```python
from build123d import *

# Parameters (mm, degrees)
ESQUISSE1_W             = 40
ESQUISSE1_H             = 27
ESQUISSE1_W_2           = 37
ESQUISSE1_H_2           = 24
BOSS_EXTRU_1_DEPTH      = 300
ESQUISSE2_R             = 2.5
ENL_V_MAT_EXTRU_1_DEPTH = 304.856874202
ESQUISSE3_R             = 6
ESQUISSE3_R_2           = 2.75
ESQUISSE3_R_3           = 10
ENL_V_MAT_EXTRU_2_DEPTH = 304.856874202


with BuildPart() as part:
    # Esquisse1 → Boss.-Extru.1 (new body)
    with BuildSketch(Plane.XY):
        with Locations((20, 13.5)):
            Rectangle(ESQUISSE1_W, ESQUISSE1_H)
        with Locations((20, 13.5)):
            Rectangle(ESQUISSE1_W_2, ESQUISSE1_H_2, mode=Mode.SUBTRACT)
    extrude(amount=BOSS_EXTRU_1_DEPTH)

    # Esquisse2 → Enlèv. mat.-Extru.1 (cut, through all)
    with BuildSketch(Plane(origin=(0, 0, 0), x_dir=(1, 0, 0), z_dir=(0, 1, 0))):
        with Locations(Location((8, -290, 0), (0, 0, 90))):
            Circle(ESQUISSE2_R)
        with Locations(Location((32, -258, 0), (0, 0, 90))):
            Circle(ESQUISSE2_R)
        with Locations(Location((7, -258, 0), (0, 0, 90))):
            Circle(ESQUISSE2_R)
        with Locations(Location((31, -290, 0), (0, 0, 90))):
            Circle(ESQUISSE2_R)
    extrude(amount=ENL_V_MAT_EXTRU_1_DEPTH, mode=Mode.SUBTRACT)

    # Esquisse3 → Enlèv. mat.-Extru.2 (cut, through all)
    with BuildSketch(Plane(origin=(0, 0, 0), x_dir=(1, 0, 0), z_dir=(0, 1, 0))):
        with Locations(Location((20, -30, 0), (0, 0, 90))):
            Circle(ESQUISSE3_R)
        with Locations(Location((5, -15, 0), (0, 0, 90))):
            Circle(ESQUISSE3_R_2)
        with Locations(Location((20, -100, 0), (0, 0, 90))):
            Circle(ESQUISSE3_R_3)
        with Locations(Location((35, -15, 0), (0, 0, 90))):
            Circle(ESQUISSE3_R_2)
        with Locations(Location((35, -45, 0), (0, 0, 90))):
            Circle(ESQUISSE3_R_2)
        with Locations(Location((5, -45, 0), (0, 0, 90))):
            Circle(ESQUISSE3_R_2)
        with Locations(Location((5, -185, 0), (0, 0, 90))):
            Circle(ESQUISSE3_R_2)
        with Locations(Location((35, -185, 0), (0, 0, 90))):
            Circle(ESQUISSE3_R_2)
        with Locations(Location((35, -155, 0), (0, 0, 90))):
            Circle(ESQUISSE3_R_2)
        with Locations(Location((20, -170, 0), (0, 0, 90))):
            Circle(ESQUISSE3_R)
        with Locations(Location((5, -155, 0), (0, 0, 90))):
            Circle(ESQUISSE3_R_2)
    extrude(amount=ENL_V_MAT_EXTRU_2_DEPTH, mode=Mode.SUBTRACT)


solid = part.part
```
The model under review builds one solid part; all positions refer to its coordinate system, in mm. A direction names the side the tool comes from. Round coordinates to 2 decimals unless told otherwise and drop trailing zeros. Write each loop counter-clockwise with the first axis right and the second up, starting at its lowest first coordinate (ties: lowest second). Pieces come first, ordered by that corner, then holes. Notation, with made-up numbers: (50.25, 66.25) -> (81.25, 66.25) arc R16 cw to (81.25, 78.25) -> close; hole circle Ø1 at (40, 67.25). An arc over 180 degrees is marked (long way). Use CSV: the item, a comma, the result in double quotes.
Q1. Consider section B-B (y = 11.5). Give the boundary of the cut face in (x, z).
Checks:
outline,"(0, 0) -> (1.5, 0) -> (1.5, 300) -> (0, 300) -> close; (38.5, 0) -> (40, 0) -> (40, 300) -> (38.5, 300) -> close"
Q2. Mouldability with a two-part tool opening along X and no side actions: class faces 3 (the cylindrical face through (32.273, 26.24, 15.358)), 4 (the flat face through (0, 13, 148)) as released by +X, released by -X, zero draft, split by the parting line, or undercut.
Checks:
face 3,"undercut"
face 4,"released by -X"
Q3. To check wall thickness, follow probe 1 along X at (y, z) = (26.65, 258); probe 2 along X at (y, z) = (26.3, 185); probe 3 along Y at (x, z) = (7, 254.5). State the ranges of each line that lie inside material, in increasing order. Write a range as [from, to].
Checks:
probe 1,"[0, 4.5], [9.5, 29.5], [34.5, 40]"
probe 2,"[0, 2.25], [7.75, 32.25], [37.75, 40]"
probe 3,"[0, 1.5], [25.5, 27]"
Q4. For pin 1 Ø5 at (x, z) = (25, 144) entering from -Y, flat-tipped, find the tip position at first contact; note if it passes through.
Checks:
pin 1,"y = 0"
Q5. Consider section A-A (z = 100). Give the boundary of the cut face in (x, y).
Checks:
outline,"(0, 0) -> (10, 0) -> (10, 1.5) -> (1.5, 1.5) -> (1.5, 25.5) -> (10, 25.5) -> (10, 27) -> (0, 27) -> close; (30, 0) -> (40, 0) -> (40, 27) -> (30, 27) -> (30, 25.5) -> (38.5, 25.5) -> (38.5, 1.5) -> (30, 1.5) -> close"
Q6. For faces 1 (the flat face through (1.5, 13, 148)), 2 (the cylindrical face through (4.17, 0.74, 182.38)), list the 3-axis set-ups (+Z, -Z, +X, -X, +Y, -Y) from which the entire face can be reached by the end or side of a thin tool; tool diameter is ignored.
Checks:
face 1,"+Z, -Z"
face 2,"+Y, -Y"
Q7. Consider section D-D (z = 15). Give the boundary of the cut face in (x, y), then the cut area to 3 significant figures.
Checks:
outline,"(0, 0) -> (2.25, 0) -> (2.25, 1.5) -> (1.5, 1.5) -> (1.5, 25.5) -> (2.25, 25.5) -> (2.25, 27) -> (0, 27) -> close; (7.75, 0) -> (32.25, 0) -> (32.25, 1.5) -> (7.75, 1.5) -> close; (7.75, 25.5) -> (32.25, 25.5) -> (32.25, 27) -> (7.75, 27) -> close; (37.75, 0) -> (40, 0) -> (40, 27) -> (37.75, 27) -> (37.75, 25.5) -> (38.5, 25.5) -> (38.5, 1.5) -> (37.75, 1.5) -> close"
area,"159 mm²"
Q8. Consider section C-C (z = 241.5). Give the boundary of the cut face in (x, y), then the cut area to 3 significant figures.
Checks:
outline,"(0, 0) -> (40, 0) -> (40, 27) -> (0, 27) -> close; hole (1.5, 1.5) -> (38.5, 1.5) -> (38.5, 25.5) -> (1.5, 25.5) -> close"
area,"192 mm²"
